Autodesk Inventor part; units mm, degrees
ref_plane "YZ Plane" through (0, 0, 0) normal (1, 0, 0) x (0, 1, 0)
ref_plane "XZ Plane" through (0, 0, 0) normal (0, 1, 0) x (-1, 0, 0)
ref_plane "XY Plane" through (0, 0, 0) normal (0, 0, 1) x (1, 0, 0)
sketch "Sketch1" plane through (0, 0, 0) normal (0, 0, 1) x (1, 0, 0)
  circle A0 centre (0, 0) radius 3.96
  dimension "d0" = 7.92
extrude "Extrusion1" add sketch "Sketch1" along normal mid plane 130.18
sketch "Sketch2" plane through (0, 0, 0) normal (0, 1, 0) x (-1, 0, 0)
  circle A0 centre (0, 56.43) radius 1.59
  line L0 (3.96, 65.09) -> (-3.96, 65.09)
  point P0 (0, 0)
  dimension "d3" = 3.18
  dimension "d4" = 8.66
extrude "Extrusion2" cut sketch "Sketch2" along normal mid plane 130.18
mirror "Mirror1" about plane through (0, 0, 0) normal (0, 0, 1) of "Extrusion2"
properties part number "parca4"
Input: part model. Units: mm. Frame: model coordinates. Coordinates: 2 decimals unless noted, no trailing zeros. Write each loop counter-clockwise with the first axis right and the second up, starting at its lowest first coordinate (ties: lowest second). Pieces come first, ordered by that corner, then holes. Notation, with made-up numbers: (7, 16.5) -> (30, 16.5) arc R26 cw to (30, 38.5) -> close; hole circle Ø7 at (-10.5, -7.5). An arc over 180 degrees is marked (long way). Write each question's results on one line, items separated by ' | '.
Item 1: Section query A-A on x = 0. Return loops of the section in (y, z), plus the area to 3 significant figures.
Conclusion:
outline: (-3.96, -65.09) -> (3.96, -65.09) -> (3.96, -58.02) -> (-3.96, -58.02) -> close; (-3.96, -54.84) -> (3.96, -54.84) -> (3.96, 54.84) -> (-3.96, 54.84) -> close; (-3.96, 58.02) -> (3.96, 58.02) -> (3.96, 65.09) -> (-3.96, 65.09) -> close | area: 981 mm^2
Item 2: Material intervals for probe 1 along Z at (x, y) = (0, 1.5); probe 2 along Z at (x, y) = (0.5, 1.5); probe 3 along Y at (x, z) = (-0.25, -36.5), sorted ascending.
Conclusion:
probe 1: z = -65.09 to -58.02, -54.84 to 54.84, 58.02 to 65.09 | probe 2: z = -65.09 to -57.94, -54.92 to 54.92, 57.94 to 65.09 | probe 3: y = -3.95 to 3.95
Item 3: Section query C-C on z = 43. Return loops of the section in (x, y), plus the area to 3 significant figures.
Conclusion:
outline: circle Ø7.92 at (0, 0) | area: 49.3 mm^2
Item 4: Section query B-B on y = 0. Return loops of the section in (x, z), plus the area to 3 significant figures.
Conclusion:
outline: (-3.96, -65.09) -> (3.96, -65.09) -> (3.96, 65.09) -> (-3.96, 65.09) -> close; hole circle Ø3.18 at (0, -56.43); hole circle Ø3.18 at (0, 56.43) | area: 1,020 mm^2
Item 5: Section query D-D on z = -56.43. Return loops of the section in (x, y), plus the area to 3 significant figures.
Conclusion:
outline: (-1.59, -3.63) -> (-1.59, 3.63) arc R3.96 ccw to start; (1.59, -3.63) arc R3.96 ccw to (1.59, 3.63) -> close | area: 24.8 mm^2
Item 6: Mould query, pull axis X, two halves, no side actions, for faces 1 (the cylindrical face through (3.658, 1.517, -0.911)), 2 (the cylindrical face through (-0.734, -0.055, -55.019)), 3 (the flat face through (0, 0, -65.09)). Classes: +X half, -X half, draft (parallel to the pull), parting line (faces both ways), or undercut.
Conclusion:
face 1: parting line | face 2: undercut | face 3: draft
Item 7: Pin query (flat end, axial travel): pin 1 Ø4 at (x, z) = (2.5, -21.5) entering from +Y; pin 2 Ø1.5 at (y, z) = (2.5, -25) entering from -X; pin 3 Ø3 at (x, z) = (1, 41.5) entering from +Y; pin 4 Ø4 at (x, z) = (3, 37.5) entering from -Y. Return the tip coordinate at first contact, or that it passes through.
Conclusion:
pin 1: stops at y = 3.93 | pin 2: stops at x = -3.55 | pin 3: stops at y = 3.96 | pin 4: stops at y = -3.83
